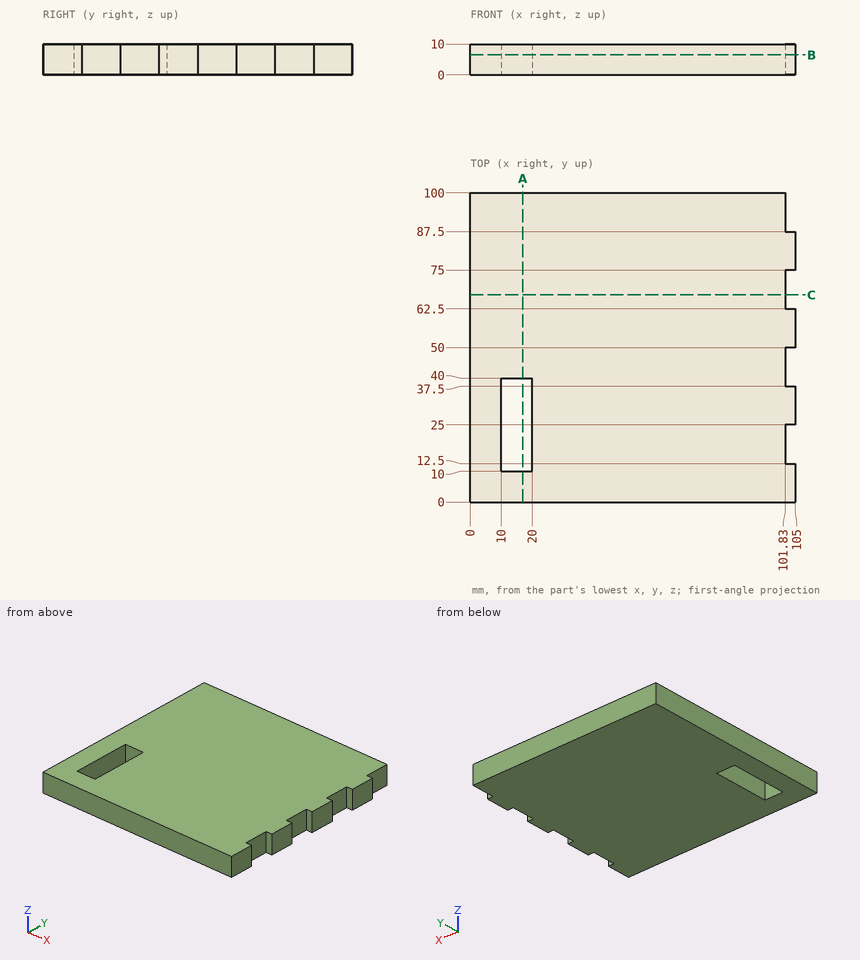
Verification items for this drawing (mm, ordinates from the low corner). Coordinates: 2 decimals unless noted, no trailing zeros. Order: outer loops, then holes, each group sorted by start corner. A loop starts at its lowest first (then second) coordinate and runs counter-clockwise, first axis right, second up. Notation, with made-up numbers: (31, 44) - (75, 44) arc R16 ccw to (75, 61) - close; hole circle Ø11 at (-19, 53.25). An arc over 180 degrees is marked (long way). Use one line per item in the form item = value.
1. Section check B-B (z = 6.5). Record the boundary of the cut face in (x, y).
Here are the results:
outline = (0, 0) - (105, 0) - (105, 12.5) - (101.83, 12.5) - (101.83, 25) - (105, 25) - (105, 37.5) - (101.83, 37.5) - (101.83, 50) - (105, 50) - (105, 62.5) - (101.83, 62.5) - (101.83, 75) - (105, 75) - (105, 87.5) - (101.83, 87.5) - (101.83, 100) - (0, 100) - close; hole (10, 10) - (20, 10) - (20, 40) - (10, 40) - close
2. Scan lines: line 1 (X direction, y = 29.5, z = 1.75); line 2 (X direction, y = 13, z = 5.5); line 3 (X direction, y = 74, z = 8.5). Record each from-to range of solid material in increasing order.
Here are the results:
line_1 = 0 to 10, 20 to 105
line_2 = 0 to 10, 20 to 101.83
line_3 = 0 to 101.83
3. Section check A-A (x = 17). Record the boundary of the cut face in (y, z), then the cut area to 3 significant figures.
Here are the results:
outline = (0, 0) - (10, 0) - (10, 10) - (0, 10) - close; (40, 0) - (100, 0) - (100, 10) - (40, 10) - close
area = 700 mm²
4. Section check C-C (y = 67). Record the boundary of the cut face in (x, z).
Here are the results:
outline = (0, 0) - (101.83, 0) - (101.83, 10) - (0, 10) - close
5. Gauge pin test, flat ends, axial feed: pin 1 (3.5 mm diameter, centred on x = 104, z = 5, fed in from +Y); pin 2 (3 mm diameter, centred on y = 67.5, z = 3.5, fed in from +X). Record the tip position at first contact, or that the pin passes through.
Here are the results:
pin_1 = 87.5
pin_2 = 101.83
